The listing builds one solid part. Answer for the finished solid, in the listing's coordinates (mm). Face numbers are marked on the shaded views. A direction names the side the tool comes from. Coordinates: 2 decimals unless noted, no trailing zeros. Order: outer loops, then holes, each group sorted by start corner. A loop starts at its lowest first (then second) coordinate and runs counter-clockwise, first axis right, second up.
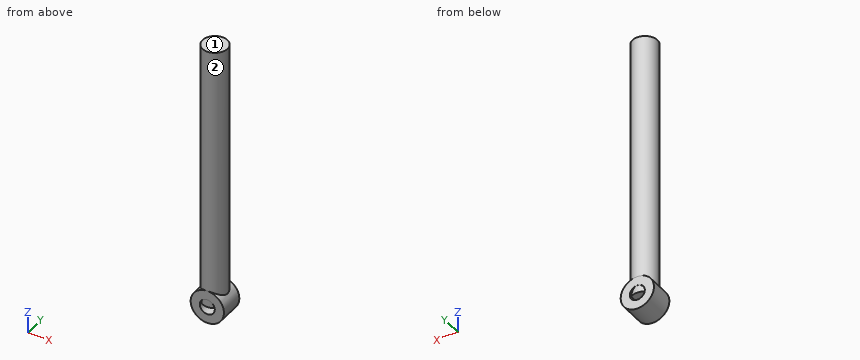
from build123d import *

# Parameters (mm, degrees)
F1_R     = 25.4
F1_R_2   = 11.43
F2_DEPTH = 19.05
F0_R     = 19.05
F3_DEPTH = 254
F4_R     = 38.1
F4_R_2   = 19.05
F5_DEPTH = 6.35
F6_DEPTH = 152.4
F7_DEPTH = 25.4


with BuildPart() as f2:
    # F1 (on Front) → F2 (new body, symmetric)
    with BuildSketch(Plane.XZ):
        Circle(F1_R)
        Circle(F1_R_2, mode=Mode.SUBTRACT)
    extrude(amount=F2_DEPTH, both=True)

    # F0 (on Top) → F3 (join)
    with BuildSketch(Plane.XY):
        Circle(F0_R)
    extrude(amount=F3_DEPTH)

    # F6 (add): a face of the model
    f6_faces = [f2.faces().sort_by_distance(p)[0] for p in [
        (0, 0, 254),
    ]]


with BuildPart() as f5:
    # F4 (on face) → F5 (new body)
    with BuildSketch(Plane.XY.offset(254)):
        Circle(F4_R)
        Circle(F4_R_2, mode=Mode.SUBTRACT)
    extrude(amount=F5_DEPTH)


with BuildPart() as f2_1:
    add(f2.part)

    add(f5.part)  # F6 merges F5
    extrude(f6_faces, amount=F6_DEPTH)

    # F7 (cut): a face of the model
    f7_faces = [f2_1.faces().sort_by_distance(p)[0] for p in [
        (-37.0223692655, 0, 260.35),
    ]]
    extrude(f7_faces, amount=-F7_DEPTH, mode=Mode.SUBTRACT)


solid = f2_1.part
(1) Given pin 1 Ø6 at (y, z) = (-10.5, 231.5) entering from +X; pin 2 Ø12 at (x, y) = (15.5, -4) entering from -Z; pin 3 Ø2 at (y, z) = (-2.5, 224) entering from +X, each flat-ended and moving along its own axis, determine where each tip first touches the part or whether it passes through.
(2) Find section A-A on y = 0. Determine the outline of the cut face in (x, z), then the cut area to 3 significant figures.
(3) Find the intervals of material crossed by probe 1 along Z at (x, y) = (0, 3); probe 2 along Z at (x, y) = (-6, 0); probe 3 along Y at (x, z) = (-0.5, 344.5), in increasing order.
(4) Find section B-B on z = 30.5. Determine the outline of the cut face in (x, y), then the cut area to 3 significant figures.
(5) A tool of negligible diameter and unlimited length cuts with its end or side. For the marked faces 1 and 2, from which of +Z, -Z, +X, -X, +Y, -Y can it reach the whole face along a straight path? Write none if from no direction.
Resolved:
1. pin 1: stops at x = 17.51
1. pin 2: stops at z = -23.56
1. pin 3: stops at x = 18.99
2. outline: (-19.05, 16.8) arc R25.4 ccw (long way) to (19.05, 16.8) - (19.05, 406.4) - (-19.05, 406.4) - close; hole (-11.43, 0) arc R11.43 ccw to (11.43, 0) - close
2. area: 16,400 mm2
3. probe 1: z = -25.4 to -11.43, 0 to 406.4
3. probe 2: z = -24.68 to -9.73, 0 to 406.4
3. probe 3: y = -19.04 to 19.04
4. outline: circle Ø38.1 at (0, 0)
4. area: 1,140 mm2
5. face 1: +Z, +X, -X, +Y, -Y
5. face 2: +Z
